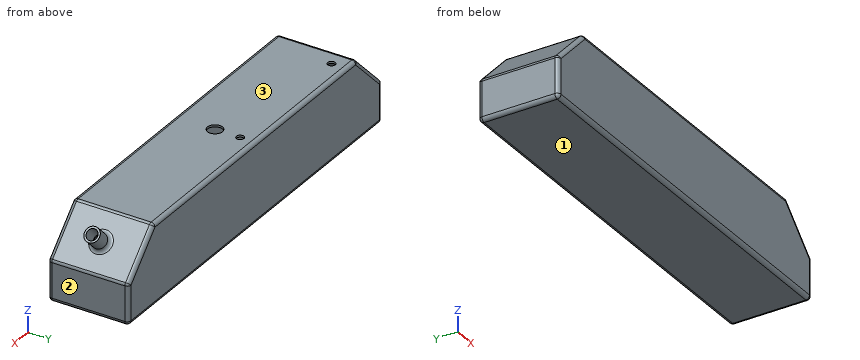
from build123d import *

# Parameters (mm, degrees)
F0_W     = 1016
F0_H     = 203.2
F1_DEPTH = 203.2
F3_DEPTH = 203.201
F4_R     = 19.05
F5_DEPTH = 50.8
F6_R     = 9.525
F7_T     = -5.08
F8_R     = 9.525
F8_R_2   = 19.05
F9_DEPTH = 5.08


with BuildPart() as f1:
    # F0 (on Top) → F1 (new body)
    with BuildSketch(Plane.XY):
        Rectangle(F0_W, F0_H)
    extrude(amount=F1_DEPTH)

    # F2 (on face) → F3 (cut, through all)
    with BuildSketch(Plane.XZ.offset(101.6)):
        Polygon((-508, 203.2), (-508, 101.6), (-406.4, 203.2), align=None)
        Polygon((508, 203.2), (406.4, 203.2), (508, 101.6), align=None)
    extrude(amount=-F3_DEPTH, mode=Mode.SUBTRACT)

    # F4 (on face) → F5 (join)
    with BuildSketch(Plane(origin=(304.8, 0, 304.8), x_dir=(0.7071067812, 0, -0.7071067812), z_dir=(0.7071067812, 0, 0.7071067812))):
        with Locations((215.5261469057, 0)):
            Circle(F4_R)
    extrude(amount=F5_DEPTH)

    # F6
    f6_edges = [f1.edges().sort_by_distance(p)[0] for p in [
        (0, -101.6, 0),
        (508, -101.6, 50.8),
        (457.2, -101.6, 152.4),
        (0, -101.6, 203.2),
        (-457.2, -101.6, 152.4),
        (-508, -101.6, 50.8),
        (406.4, 0, 203.2),
        (508, 0, 101.6),
        (457.2, 101.6, 152.4),
        (443.729616, 0, 165.870384),
        (508, 0, 0),
        (508, 101.6, 50.8),
        (-406.4, 0, 203.2),
        (0, 101.6, 203.2),
        (-508, 0, 0),
        (-508, 0, 101.6),
        (-508, 101.6, 50.8),
        (-457.2, 101.6, 152.4),
        (0, 101.6, 0),
    ]]
    fillet(f6_edges, radius=F6_R)

    # F7
    f7_openings = [f1.faces().sort_by_distance(p)[0] for p in [
        (493.121024, 0, 188.321024),
    ]]
    offset(amount=F7_T, openings=f7_openings)

    # F8 (on face) → F9 (cut)
    with BuildSketch(Plane.XY.offset(203.2)):
        with Locations((-366.3365542889, 63.5)):
            Circle(F8_R)
        with Locations((0, 63.5)):
            Circle(F8_R)
        Circle(F8_R_2)
    extrude(amount=-F9_DEPTH, mode=Mode.SUBTRACT)


solid = f1.part
The listing builds one solid part. Answer for the finished solid, in the listing's coordinates (mm). Face numbers are marked on the shaded views. Give positions to 0.01 mm unless a question says otherwise; leave off trailing zeros. Write each loop counter-clockwise with the first axis right and the second up, starting at its lowest first coordinate (ties: lowest second). Pieces come first, ordered by that corner, then holes.
1) Section B-B (x = -95) is taken. Write down the section's boundary in (y, z) (3 decimals), and give its area (3 significant figures).
2) Section A-A (z = 18) is taken. Write down the section's boundary in (x, y) (3 decimals).
3) For a pull along Z with two mould halves and no side action, classify the marked faces 1, 2 and 3 as pulls with the +Z half, pulls with the -Z half, needs draft (parallel to the pull), parting line crosses it, or undercut.
4) Section C-C (y = 43.5) is taken. Write down the section's boundary in (x, z) (3 decimals), and give its area (3 significant figures).
5) Find the intervals of material crossed by L1, parallel to Y at x = 458.5, z = 136; L2, parallel to Z at x = -90, y = 87; L3, parallel to Y at x = 0, z = 200.85 (3 decimals), in increasing order.
Response:
1. outline: (-101.6, 9.525) arc R9.525 ccw to (-92.075, 0) - (92.075, 0) arc R9.525 ccw to (101.6, 9.525) - (101.6, 193.675) arc R9.525 ccw to (92.075, 203.2) - (-92.075, 203.2) arc R9.525 ccw to (-101.6, 193.675) - close; hole (-96.52, 9.525) arc R4.445 ccw to (-92.075, 5.08) - (92.075, 5.08) arc R4.445 ccw to (96.52, 9.525) - (96.52, 193.675) arc R4.445 ccw to (92.075, 198.12) - (-92.075, 198.12) arc R4.445 ccw to (-96.52, 193.675) - close
1. area: 3,960 mm2
2. outline: (-508, -92.075) arc R9.525 ccw to (-498.475, -101.6) - (498.475, -101.6) arc R9.525 ccw to (508, -92.075) - (508, 92.075) arc R9.525 ccw to (498.475, 101.6) - (-498.475, 101.6) arc R9.525 ccw to (-508, 92.075) - close; hole (-502.92, -92.075) arc R4.445 ccw to (-498.475, -96.52) - (498.475, -96.52) arc R4.445 ccw to (502.92, -92.075) - (502.92, 92.075) arc R4.445 ccw to (498.475, 96.52) - (-498.475, 96.52) arc R4.445 ccw to (-502.92, 92.075) - close
3. face 1: pulls with the -Z half
3. face 2: needs draft
3. face 3: pulls with the +Z half
4. outline: (-508, 9.525) arc R9.525 ccw to (-498.475, 0) - (498.475, 0) arc R9.525 ccw to (508, 9.525) - (508, 97.655) arc R9.525 ccw to (505.21, 104.39) - (409.19, 200.41) arc R9.525 ccw to (402.455, 203.2) - (-402.455, 203.2) arc R9.525 ccw to (-409.19, 200.41) - (-505.21, 104.39) arc R9.525 ccw to (-508, 97.655) - close; hole (-502.92, 9.525) arc R4.445 ccw to (-498.475, 5.08) - (498.475, 5.08) arc R4.445 ccw to (502.92, 9.525) - (502.92, 97.655) arc R4.445 ccw to (501.618, 100.798) - (405.598, 196.818) arc R4.445 ccw to (402.455, 198.12) - (-402.455, 198.12) arc R4.445 ccw to (-405.598, 196.818) - (-501.618, 100.798) arc R4.445 ccw to (-502.92, 97.655) - close
4. area: 11,700 mm2
5. L1: y = -101.6 to -96.52, 96.52 to 101.6
5. L2: z = 0 to 5.08, 198.12 to 203.2
5. L3: y = -98.34 to -19.05, 19.05 to 53.975, 73.025 to 98.34
